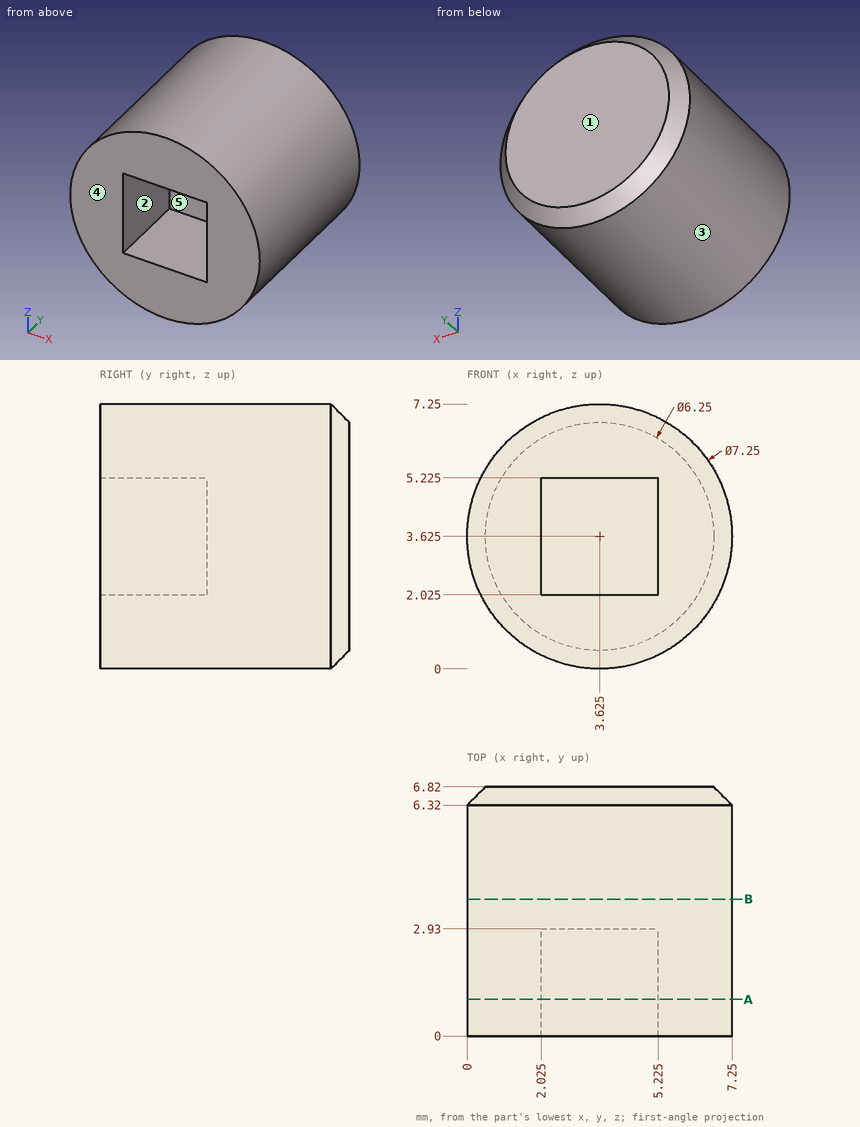
Part print with two shaded views. Sizes in mm from the minimum x, y, z corner. A direction names the side the tool comes from. Coordinates: 2 decimals unless noted, no trailing zeros. Order: outer loops, then holes, each group sorted by start corner. A loop starts at its lowest first (then second) coordinate and runs counter-clockwise, first axis right, second up. Notation, with made-up numbers: (33, -25.5) - (81, -25.5) arc R16 ccw to (81, -18.5) - close; hole circle Ø7 at (48, 45.25). An arc over 180 degrees is marked (long way). Answer in a Markdown table with one row per item.
1. Flat gauge pins, fed straight in: P1, Ø1.5, axis at y = 1, z = 4, coming from the -X side; P2, Ø0.9, axis at y = 1, z = 3, coming from the +X side; P3, Ø0.9, axis at x = 3, y = 2, coming from the -Z side; P4, Ø1.6, axis at x = 4, z = 3, coming from the -Y side. Where does each tip first touch, or does it go through?
Answer:
| item | result |
|---|---|
| P1 | x = 0 |
| P2 | x = 7.25 |
| P3 | z = 0 |
| P4 | y = 2.93 |
2. Drill centre lines: L1, parallel to Z at x = 3.75, y = 0.75 (3 decimals); L2, parallel to Y at x = 5, z = 2.25; L3, parallel to Z at x = 3.5, y = 6.25. Where is each one in solid material? Low to high. Write a range as from..to.
Answer:
| item | result |
|---|---|
| L1 | 0.002..2.025, 5.225..7.248 |
| L2 | 2.93..6.82 |
| L3 | 0..7.25 |
3. 3-axis set-ups, long thin cutter, end or side, ignore diameter. For the marked faces 4 and 5: which of +Z, -Z, +X, -X, +Y, -Y reach the whole face in a straight line?
Answer:
| item | result |
|---|---|
| face 4 | +Z, -Z, +X, -X, -Y |
| face 5 | -Y |
4. Pull direction X, two halves, no side cores. Call the marked faces 1, 2 and 3: +X half, -X half, draft (parallel to the pull), parting line (faces both ways), or undercut.
Answer:
| item | result |
|---|---|
| face 1 | draft |
| face 2 | undercut |
| face 3 | parting line |
5. Slice it at B-B, the plane y = 3.75. List the corners of the cut face in (x, z) (3 decimals).
Answer:
| item | result |
|---|---|
| outline | circle Ø7.25 at (3.625, 3.625) |
6. Slice it at A-A, the plane y = 1. List the corners of the cut face in (x, z) (3 decimals).
Answer:
| item | result |
|---|---|
| outline | circle Ø7.25 at (3.625, 3.625); hole (2.025, 2.025) - (5.225, 2.025) - (5.225, 5.225) - (2.025, 5.225) - close |
